from build123d import *

# Parameters (mm, degrees)
CROQUIS1_W              = 85
CROQUIS1_H              = 30
CROQUIS1_W_2            = 16
CROQUIS1_H_2            = 23
SALIENTE_EXTRUIR1_DEPTH = 3
CROQUIS3_W              = 30
CROQUIS3_H              = 30
SALIENTE_EXTRUIR2_DEPTH = 10


with BuildPart() as part:
    # Croquis1 → Saliente-Extruir1 (new body)
    with BuildSketch(Plane(origin=(0, 0, 0), x_dir=(1, 0, 0), z_dir=(0, 1, 0))):
        Rectangle(CROQUIS1_W, CROQUIS1_H)
        with Locations((30, 0)):
            Rectangle(CROQUIS1_W_2, CROQUIS1_H_2, mode=Mode.SUBTRACT)
        with Locations((-30, 0)):
            Rectangle(CROQUIS1_W_2, CROQUIS1_H_2, mode=Mode.SUBTRACT)
    extrude(amount=SALIENTE_EXTRUIR1_DEPTH)

    # Croquis3 → Saliente-Extruir2 (add)
    with BuildSketch(Plane(origin=(0, 3, 0), x_dir=(1, 0, 0), z_dir=(0, 1, 0))):
        Rectangle(CROQUIS3_W, CROQUIS3_H)
    extrude(amount=SALIENTE_EXTRUIR2_DEPTH)


solid = part.part
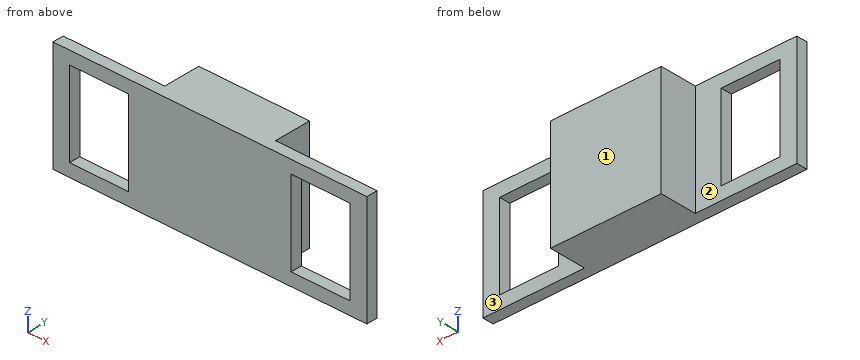
Part model, mm, in its own coordinate system. Face numbers are marked on the shaded views. A direction names the side the tool comes from. Round coordinates to 2 decimals unless told otherwise and drop trailing zeros. Write each loop counter-clockwise with the first axis right and the second up, starting at its lowest first coordinate (ties: lowest second). Pieces come first, ordered by that corner, then holes. Notation, with made-up numbers: (-15, -35.75) - (-11, -35.75) arc R24 ccw to (-11, -18.75) - close; hole circle Ø6 at (78, -16.75). An arc over 180 degrees is marked (long way). Use CSV: the item, a comma, the result in double quotes.
Item 1: Slice it at D-D, the plane y = 12.25. Write the cut outline in (x, z), then the cut area to 3 significant figures.
Results list:
outline,"(-15, -15) - (15, -15) - (15, 15) - (-15, 15) - close"
area,"900 mm²"
Item 2: Wall check: L1, parallel to X at y = 1, z = -10.5; L2, parallel to X at y = 6.25, z = -13; L3, parallel to Y at x = -35.5, z = 12.5. Give the ranges that are in metal, low to high.
Results list:
L1,"x = -42.5 to -38, -22 to 22, 38 to 42.5"
L2,"x = -15 to 15"
L3,"y = 0 to 3"
Item 3: Tool access for the marked faces 1, 2 and 3: list every direction of +Z, -Z, +X, -X, +Y, -Y with a clear straight run to the whole face (end or side of a thin tool).
Results list:
face 1,"+Z, -Z, +X, -X, +Y"
face 2,"+Z, -Z, -X, +Y"
face 3,"+Z, -Z, +X, +Y"
Item 4: Slice it at B-B, the plane x = -37. Write the cut outline in (y, z).
Results list:
outline,"(0, -15) - (3, -15) - (3, -11.5) - (0, -11.5) - close; (0, 11.5) - (3, 11.5) - (3, 15) - (0, 15) - close"
Item 5: Slice it at A-A, the plane y = 2. Write the cut outline in (x, z).
Results list:
outline,"(-42.5, -15) - (42.5, -15) - (42.5, 15) - (-42.5, 15) - close; hole (-38, -11.5) - (-22, -11.5) - (-22, 11.5) - (-38, 11.5) - close; hole (22, -11.5) - (38, -11.5) - (38, 11.5) - (22, 11.5) - close"
Item 6: Flat gauge pins, fed straight in: P1, Ø4, axis at y = 6.5, z = 2.5, coming from the +X side; P2, Ø5, axis at y = 6.5, z = -3.5, coming from the -X side. Where does each tip first touch, or does it go through?
Results list:
P1,"stops at x = 15"
P2,"stops at x = -15"
Item 7: Slice it at C-C, the plane z = -2. Write the cut outline in (x, y).
Results list:
outline,"(-42.5, 0) - (-38, 0) - (-38, 3) - (-42.5, 3) - close; (-22, 0) - (22, 0) - (22, 3) - (15, 3) - (15, 13) - (-15, 13) - (-15, 3) - (-22, 3) - close; (38, 0) - (42.5, 0) - (42.5, 3) - (38, 3) - close"
